Autodesk Inventor part; units mm, degrees
ref_plane "YZ Plane" through (0, 0, 0) normal (1, 0, 0) x (0, 1, 0)
ref_plane "XZ Plane" through (0, 0, 0) normal (0, 1, 0) x (-1, 0, 0)
ref_plane "XY Plane" through (0, 0, 0) normal (0, 0, 1) x (1, 0, 0)
sketch "Sketch1" plane through (0, 0, 0) normal (1, 0, 0) x (0, 1, 0)
  line L0 (38.1, 101.6) -> (-38.1, 101.6)
  line L1 (-38.1, 101.6) -> (-38.1, -101.6)
  line L2 (-38.1, -101.6) -> (38.1, -101.6)
  line L3 (38.1, -101.6) -> (38.1, 101.6)
  line L4 (38.1, 101.6) -> (-38.1, -101.6) construction
  line L5 (-38.1, 101.6) -> (38.1, -101.6) construction
  point P0 (0, 0)
  dimension "d0" = 76.2
  dimension "d1" = 203.2
extrude "Extrusion1" add sketch "Sketch1" along normal mid plane 50.8
sketch "Sketch2" plane through (-25.4, 38.1, 101.6) normal (0, 1, 0) x (1, 0, 0)
  line L0 (4, 199.2) -> (46.8, 199.2)
  line L1 (46.8, 199.2) -> (46.8, 4)
  line L2 (46.8, 4) -> (4, 4)
  line L3 (4, 4) -> (4, 199.2)
  line L4 (4, 199.2) -> (46.8, 4) construction
  line L5 (46.8, 199.2) -> (4, 4) construction
  line L6 (0, 0) -> (0, 203.2)
  line L7 (0, 0) -> (50.8, 0)
  point P0 (25.4, 101.6)
  dimension "d4" = 4
  dimension "d5" = 4
extrude "Extrusion2" cut sketch "Sketch2" against normal blind 47.8
sketch "Sketch5" plane through (-25.4, -38.1, -101.6) normal (0, -1, 0) x (1, 0, 0)
  circle A0 centre (25.4, 152.4) radius 2
  circle A1 centre (25.4, 177.8) radius 2
  circle A2 centre (25.4, 50.8) radius 2
  circle A3 centre (25.4, 25.4) radius 2
  line L0 (50.8, 203.2) -> (0, 203.2)
  line L1 (0, 0) -> (50.8, 0)
  line L2 (50.8, 203.2) -> (50.8, 0)
  point P0 (25.4, 101.6)
  dimension "d33" = 4
  dimension "d34" = 4
  dimension "d35" = 4
  dimension "d36" = 4
  dimension "d37" = 25.4
  dimension "d38" = 25.4
  dimension "d39" = 50.8
  dimension "d40" = 50.8
  dimension "d41" = 25.4
  dimension "d42" = 25.4
  dimension "d43" = 25.4
  dimension "d44" = 25.4
extrude "Extrusion5" cut sketch "Sketch5" against normal through all
sketch "Sketch6" plane through (25.4, 0, 0) normal (1, 0, 0) x (0, 0, -1)
  point P0 (0, 0)
sketch "Sketch7" plane through (25.4, 0, 0) normal (1, 0, 0) x (0, 0, -1)
  point P0 (0, 0)
sketch "Sketch8" plane through (25.4, 0, 0) normal (1, 0, 0) x (0, 0, -1)
  circle A0 centre (-69.85, 12.7) radius 5
  circle A1 centre (-31.75, 12.7) radius 5
  circle A2 centre (31.75, 12.7) radius 5
  circle A3 centre (69.85, 12.7) radius 5
  line L0 (-101.6, 38.1) -> (-101.6, -38.1)
  line L1 (101.6, -38.1) -> (101.6, 38.1)
  line L2 (101.6, 38.1) -> (-101.6, 38.1)
  point P0 (0, 0)
  dimension "d47" = 10
  dimension "d48" = 10
  dimension "d49" = 10
  dimension "d50" = 10
  dimension "d51" = 31.75
  dimension "d52" = 69.85
  dimension "d53" = 31.75
  dimension "d54" = 69.85
  dimension "d55" = 25.4
  dimension "d56" = 25.4
  dimension "d57" = 25.4
  dimension "d58" = 25.4
sketch "Sketch9" plane through (25.4, 0, 0) normal (1, 0, 0) x (0, 0, -1)
  point P0 (0, 0)
sketch "Sketch10" plane through (25.4, 0, 0) normal (1, 0, 0) x (0, 0, -1)
  point P0 (0, 0)
extrude "Extrusion6" cut sketch "Sketch8" against normal through all
fillet "Fillet1" radius 2 13 edges at (0, 38.1, 101.6) (0, 38.1, 97.6) (-21.4, 12.7, 74.85) (25.4, 38.1, 0) (21.4, 38.1, 0) (-21.4, 38.1, 0) (-25.4, 38.1, 0) (0, 38.1, -97.6) (0, 38.1, -101.6) (25.4, 0, 101.6) (-25.4, 0, 101.6) (25.4, 0, -101.6) (-25.4, 0, -101.6)
sketch "Sketch11" plane through (0, 0, 0) normal (0, 1, 0) x (-1, 0, 0)
  point P0 (0, 0)
sketch "Sketch12" plane through (0, 0, 0) normal (0, 1, 0) x (-1, 0, 0)
  point P0 (0, 0)
sketch "Sketch13" plane through (-25.4, 0, 0) normal (-1, 0, 0) x (0, 0, 1)
  circle A0 centre (0, 12.7) radius 5
  line L0 (-99.6, -38.1) -> (99.6, -38.1)
  point P0 (0, 0)
  dimension "d62" = 10
  dimension "d63" = 50.8
extrude "Extrusion7" cut sketch "Sketch13" against normal blind 4
sketch "Sketch14" plane through (25.4, 0, 0) normal (1, 0, 0) x (0, 0, -1)
  circle A0 centre (0, 12.7) radius 17.5
  line L0 (-99.6, 36.1) -> (99.6, 36.1)
  point P0 (0, 0)
  dimension "d66" = 35
  dimension "d69" = 23.4
extrude "Extrusion8" cut sketch "Sketch14" against normal blind 4
sketch "Sketch15" plane through (25.4, 0, 0) normal (1, 0, 0) x (0, 0, -1)
  point P0 (0, 0)
properties part number "gear holder" material "Stainless Steel"
Design review of the part built by this model. Coordinates are the model's own, in mm. A direction names the side the tool comes from. Give positions to 0.01 mm unless a question says otherwise; leave off trailing zeros. Write item = value, one per line. Start each with the question number.
(1) For faces 5 (the face through (0, 14, 97.6)), 6 (the face through (23.428, 16.079, 35.435)), list the 3-axis set-ups (+Z, -Z, +X, -X, +Y, -Y) from which the entire face can be reached by the end or side of a thin tool; tool diameter is ignored.
(2) We need section A-A on x = 0. State how many separate pieces and enclosed holes the cut face has, plus the area to 3 significant figures.
(3) For pin 1 (2 mm diameter, centred on x = -9, z = 26, fed in from +Y), flat-tipped, find the tip position at first contact; note if it passes through.
(4) To check wall thickness, follow line 1 along Z through (x, y) = (0, -16.25); line 2 along X through (y, z) = (23, -73); line 3 along Z through (x, y) = (-22, 12). State the ranges of each line that lie inside material, in increasing order.
(5) Mouldability with a two-part tool opening along Y and no side actions: class faces 1 (the face through (23.428, 12.92, -26.755)), 2 (the face through (-23.372, 12.92, -26.755)), 3 (the face through (25.4, -10, 1)), 4 (the face through (0, -9.7, -1)) as +Y half, -Y half, draft (parallel to the pull), parting line (faces both ways), or undercut.
Numbers:
q1.face_5 = +Y
q1.face_6 = +X, -X
q2.separate_pieces = 5
q2.enclosed_holes = 0
q2.area = 5,700 mm^2
q3.pin_1 = -9.7
q4.line_1 = -101.6 to -78.2, -74.2 to -52.8, -48.8 to 48.8, 52.8 to 74.2, 78.2 to 101.6
q4.line_2 = -25.4 to -21.4, 21.4 to 25.4
q4.line_3 = -101.6 to -74.8, -64.9 to -36.7, -26.8 to -4.95, 4.95 to 26.8, 36.7 to 64.32, 75.38 to 101.6
q5.face_1 = undercut
q5.face_2 = undercut
q5.face_3 = draft
q5.face_4 = +Y half
